Could you check a few things on this drawing? It's one solid part, dimensions in mm from its lowest x, y, z. Give positions to 0.01 mm unless a question says otherwise; leave off trailing zeros. Loops run counter-clockwise (first coordinate to the right, second up) from the corner with the lowest first, then second, coordinate; pieces in that order, holes last.
1. Imagine slicing it at C-C (z = 37.5). List the corners of the cut face in (x, y) for me (1 decimal).
2. Imagine slicing it at A-A (z = 5). List the corners of the cut face in (x, y) for me (1 decimal), plus the area to 3 significant figures.
3. For P1, Ø4, axis at y = 10, z = 29, coming from the -X side; P2, Ø6, axis at x = 37.5, z = 15.5, coming from the +Y side, each with a flat end and sliding along its axis, tell me the tip position at first contact or that it passes through.
4. Imagine slicing it at D-D (y = 3.75). List the corners of the cut face in (x, z) for me.
5. Thinking about a two-plate mould opening in X: for the marked faces 1, 2 and 3, which applies, +X half, -X half, draft (parallel to the pull), parting line (faces both ways), or undercut?
6. I need wall thicknesses on line 1 along Y through (x, z) = (34.5, 9); line 2 along X through (y, z) = (13.25, 47.5) (1 decimal); line 3 along X through (y, z) = (4, 3) (1 decimal). Which ranges of each line are inside material? Lowest first, please.
7. Imagine slicing it at B-B (y = 13). List the corners of the cut face in (x, z) for me, plus the area to 3 significant figures.
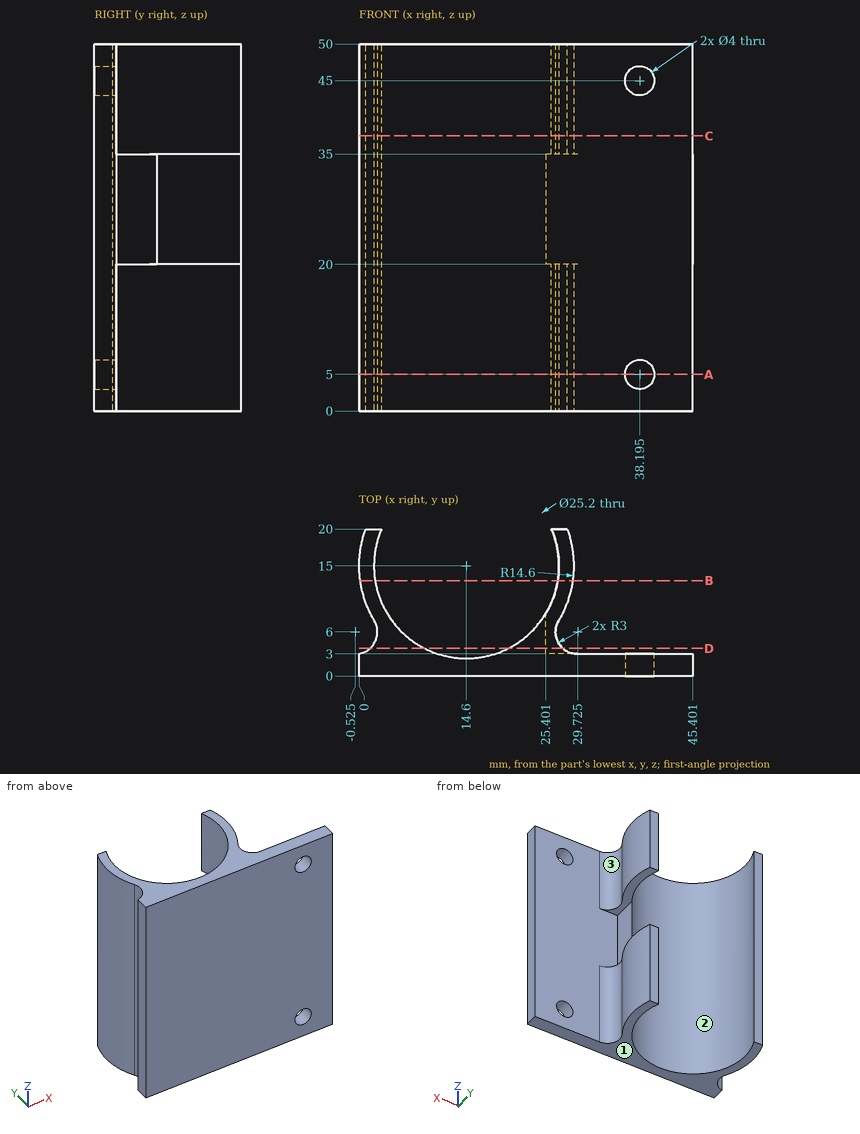
Derived:
1. outline: (0, 0) - (45.4, 0) - (45.4, 3) - (29.7, 3) arc R3 cw to (27.1, 7.5) arc R14.6 ccw to (28.3, 20) - (26.2, 20) arc R12.6 cw (long way) to (3, 20) - (0.9, 20) arc R14.6 ccw to (2.1, 7.5) arc R3 cw to (0, 3) - close
2. outline: (0, 0) - (36.2, 0) - (36.2, 3) - (29.7, 3) arc R3 cw to (27.1, 7.5) arc R14.6 ccw to (28.3, 20) - (26.2, 20) arc R12.6 cw (long way) to (3, 20) - (0.9, 20) arc R14.6 ccw to (2.1, 7.5) arc R3 cw to (0, 3) - close; (40.2, 0) - (45.4, 0) - (45.4, 3) - (40.2, 3) - close
2. area: 218 mm2
3. P1: stops at x = 0.31
3. P2: stops at y = 3
4. outline: (1.46, 0) - (8.93, 0) - (8.93, 50) - (1.46, 50) - close; (20.27, 0) - (27.74, 0) - (27.74, 20) - (25.4, 20) - (25.4, 35) - (27.74, 35) - (27.74, 50) - (20.27, 50) - close
5. face 1: draft
5. face 2: undercut
5. face 3: +X half
6. line 1: y = 0 to 3
6. line 2: x = 0.1 to 2.1, 27.1 to 29.1
6. line 3: x = 1.7 to 8.5, 20.7 to 27.5
7. outline: (0.14, 0) - (2.16, 0) - (2.16, 50) - (0.14, 50) - close; (27.04, 0) - (29.06, 0) - (29.06, 20) - (27.04, 20) - close; (27.04, 35) - (29.06, 35) - (29.06, 50) - (27.04, 50) - close
7. area: 172 mm2
